```python
from build123d import *

# Parameters (mm, degrees)
CUT_EXTRUDE1_DEPTH = 7.35


with BuildPart() as part:
    # Sketch1 → Revolve1 (revolve)
    with BuildSketch(Plane(origin=(0, 0, 0), x_dir=(0, 0, -1), z_dir=(1, 0, 0))):
        Polygon((74.67454347, 0), (76.2, 2.210784201), (76.2, 3.175), (0, 3.175), (0, -3.175), (76.2, -3.175), (76.2, -2.210784201), align=None)
    revolve(axis=Axis((0, -3.175, 0), (0, 1, 0)))

    # Sketch2 → Cut-Extrude1 (cut, through all)
    with BuildSketch(Plane(origin=(0, 3.175, 0), x_dir=(1, 0, 0), z_dir=(0, 1, 0))):
        with BuildLine():
            Line((-3.110851973, 3.175), (3.110851973, 3.175))
            ThreePointArc((3.110851973, 3.175), (4.445, 0), (3.110851973, -3.175))
            Line((3.110851973, -3.175), (-3.110851973, -3.175))
            ThreePointArc((-3.110851973, -3.175), (-4.445, 0), (-3.110851973, 3.175))
        make_face()
        with BuildLine():
            Line((-17.302740061, 33.589551898), (4.896011221, 60.125990213))
            ThreePointArc((4.896011221, 60.125990213), (20.500009374, 56.734956073), (34.667618402, 49.368632342))
            Line((34.667618402, 49.368632342), (4.035924256, 33.589551898))
            Line((4.035924256, 33.589551898), (1.51506049, 12.609305759))
            ThreePointArc((1.51506049, 12.609305759), (-2.249253525, 12.49923432), (-5.815791429, 11.290109391))
            Line((-5.815791429, 11.290109391), (-17.302740061, 33.589551898))
        make_face()
        with BuildLine():
            Line((15.473287184, 34.470569971), (50.061005129, 33.660086013))
            ThreePointArc((50.061005129, 33.660086013), (57.138721597, 19.346113801), (60.21285754, 3.676603308))
            Line((60.21285754, 3.676603308), (28.777726771, 17.787330414))
            Line((28.777726771, 17.787330414), (10.802976979, 6.67725156))
            ThreePointArc((10.802976979, 6.67725156), (8.369908264, 9.551682347), (5.200876316, 11.586236902))
            Line((5.200876316, 11.586236902), (15.473287184, 34.470569971))
        make_face()
        with BuildLine():
            Line((36.597613582, 9.394545783), (57.529041117, -18.152549495))
            ThreePointArc((57.529041117, -18.152549495), (50.75081104, -32.610746752), (40.416586831, -44.783983006))
            Line((40.416586831, -44.783983006), (31.849314069, -11.409113668))
            Line((31.849314069, -11.409113668), (11.956031462, -4.282909254))
            ThreePointArc((11.956031462, -4.282909254), (12.686358414, -0.588481252), (12.301178117, 3.15769171))
            Line((12.301178117, 3.15769171), (36.597613582, 9.394545783))
        make_face()
        with BuildLine():
            Line((30.163190498, -22.755762993), (21.676535765, -56.295944989))
            ThreePointArc((21.676535765, -56.295944989), (6.146504642, -60.011049863), (-9.814198109, -59.52131669))
            Line((-9.814198109, -59.52131669), (10.937718265, -32.014262454))
            Line((10.937718265, -32.014262454), (4.105950396, -12.017952045))
            ThreePointArc((4.105950396, -12.017952045), (7.449721924, -10.285506465), (10.138441898, -7.648659745))
            Line((10.138441898, -7.648659745), (30.163190498, -22.755762993))
        make_face()
        with BuildLine():
            Line((1.015269752, -37.770518102), (-30.498843139, -52.047345679))
            ThreePointArc((-30.498843139, -52.047345679), (-43.086245118, -42.221808425), (-52.6546917, -29.437884892))
            Line((-52.6546917, -29.437884892), (-18.210202481, -28.512018641))
            Line((-18.210202481, -28.512018641), (-6.835995065, -10.703231824))
            ThreePointArc((-6.835995065, -10.703231824), (-3.396707121, -12.237335524), (0.341252143, -12.695414407))
            Line((0.341252143, -12.695414407), (1.015269752, -37.770518102))
        make_face()
        with BuildLine():
            Line((-28.897169825, -24.343302703), (-59.707971096, -8.606033499))
            ThreePointArc((-59.707971096, -8.606033499), (-59.874173504, 7.361315925), (-55.845128481, 22.812874653))
            Line((-55.845128481, 22.812874653), (-33.645469338, -3.539643251))
            Line((-33.645469338, -3.539643251), (-12.630296812, -1.328759734))
            ThreePointArc((-12.630296812, -1.328759734), (-11.685346424, -4.974201337), (-9.712907436, -8.182263082))
            Line((-9.712907436, -8.182263082), (-28.897169825, -24.343302703))
        make_face()
        with BuildLine():
            Line((-37.049451129, 7.414916145), (-43.955778997, 41.315797436))
            ThreePointArc((-43.955778997, 41.315797436), (-31.575628032, 51.40121924), (-16.983044483, 57.885074286))
            Line((-16.983044483, 57.885074286), (-23.745011542, 24.098155702))
            Line((-23.745011542, 24.098155702), (-8.913727449, 9.046295538))
            ThreePointArc((-8.913727449, 9.046295538), (-11.174681532, 6.034607912), (-12.453049608, 2.492299232))
            Line((-12.453049608, 2.492299232), (-37.049451129, 7.414916145))
        make_face()
    extrude(amount=-CUT_EXTRUDE1_DEPTH, mode=Mode.SUBTRACT)


solid = part.part
```
Geometry check sheet. Reference: the model listing, model coordinates, mm. Coordinates: 2 decimals unless noted, no trailing zeros. Put each result on its own line as item: value.
1) Gauge pin test, flat ends, axial feed: pin 1 Ø1.9 at (x, y) = (0.5, -1) entering from -Z; pin 2 Ø2 at (y, z) = (0.5, -31) entering from -X; pin 3 Ø1.9 at (x, y) = (0.5, 0) entering from +Z. Record the tip position at first contact, or that the pin passes through.
Result set:
pin 1: stops at z = -76.02
pin 2: stops at x = -69.19
pin 3: stops at z = 75.33
2) Cross-section at A-A on x = -21. Count the separate pieces of the cut face and the enclosed holes in it, plus the area to 3 significant figures.
Result set:
separate pieces: 5
enclosed holes: 0
area: 476 mm^2
3) Release check for a two-part mould opening along Y. For faces 1 (the flat face through (-11.479, 0.044, -22.284)), 2 (the conical face through (72.992, 0.138, 16.209)) record: released by +Y, released by -Y, zero draft, split by the parting line, or undercut.
Result set:
face 1: zero draft
face 2: undercut
4) Thickness scan on line 1 (X direction, y = -0.25, z = 41.5); line 2 (Z direction, x = 45.5, y = 1.5); line 3 (X direction, y = -2.75, z = 24.5). Record the ranges inside material, lowest first.
Result set:
line 1: x = -62.29 to -43.78, -7.22 to 3.78, 25.42 to 39.57, 43.78 to 62.29
line 2: z = -60.51 to -33.77, -10.28 to 2.32, 39.61 to 60.51
line 3: x = -72.15 to -15.65, 0.66 to 8.37, 29.72 to 35.21, 55.13 to 72.15
